from build123d import *

# Parameters (mm, degrees)
F0_R      = 2.7305
F1_DEPTH  = 13.716
F0_W      = 71.12
F0_H      = 39.37
F0_H_2    = 6.35
F2_DEPTH  = 5.08
F3_DEPTH  = 25.4
F4_W      = 43.18
F4_H      = 25.4
F5_DEPTH  = 6.351
F6_R      = 1
F7_DEPTH  = 9
F8_R      = 5.08
F9_W      = 48
F9_H      = 17
F9_W_2    = 11
F9_H_2    = 6.2
F10_DEPTH = 25.4


with BuildPart() as f1:
    # F0 (on Front) → F1 (new body)
    with BuildSketch(Plane.XZ):
        with Locations((6.9215, 40.386)):
            Circle(F0_R)
    extrude(amount=F1_DEPTH)



with BuildPart() as f1b:
    # F0 (on Front) → F1, piece 2 (new body)
    with BuildSketch(Plane.XZ):
        with Locations((6.9215, 10.668)):
            Circle(F0_R)
    extrude(amount=F1_DEPTH)


with BuildPart() as f1c:
    # F0 (on Front) → F1, piece 3 (new body)
    with BuildSketch(Plane.XZ):
        with Locations((64.1985, 10.668)):
            Circle(F0_R)
    extrude(amount=F1_DEPTH)


with BuildPart() as f1d:
    # F0 (on Front) → F1, piece 4 (new body)
    with BuildSketch(Plane.XZ):
        with Locations((64.1985, 40.386)):
            Circle(F0_R)
    extrude(amount=F1_DEPTH)


with BuildPart() as f1_1:
    add(f1.part)

    add(f1b.part)  # F2 merges F1b

    add(f1c.part)  # F2 merges F1c

    add(f1d.part)  # F2 merges F1d
    # F0 (on Front) → F2 (join)
    with BuildSketch(Plane.XZ):
        with Locations((35.56, 26.035)):
            Rectangle(F0_W, F0_H)
        with Locations((6.9215, 10.668)):
            Circle(F0_R, mode=Mode.SUBTRACT)
        with Locations((64.1985, 10.668)):
            Circle(F0_R, mode=Mode.SUBTRACT)
        with Locations((6.9215, 40.386)):
            Circle(F0_R, mode=Mode.SUBTRACT)
        with Locations((64.1985, 40.386)):
            Circle(F0_R, mode=Mode.SUBTRACT)
        with Locations((35.56, 3.175)):
            Rectangle(F0_W, F0_H_2)
        with Locations((64.1985, 40.386)):
            Circle(F0_R)
        with Locations((6.9215, 40.386)):
            Circle(F0_R)
        with Locations((6.9215, 10.668)):
            Circle(F0_R)
        with Locations((64.1985, 10.668)):
            Circle(F0_R)
    extrude(amount=-F2_DEPTH)

    # F0 (on Front) → F3 (join)
    with BuildSketch(Plane.XZ):
        with Locations((35.56, 3.175)):
            Rectangle(F0_W, F0_H_2)
    extrude(amount=F3_DEPTH)

    # F4 (on face) → F5 (cut, through all)
    with BuildSketch(Plane.XY.offset(6.35)):
        with Locations((35.56, -12.7)):
            Rectangle(F4_W, F4_H)
    extrude(amount=-F5_DEPTH, mode=Mode.SUBTRACT)

    # F6 (on face) → F7 (cut)
    with BuildSketch(Plane.XZ.offset(13.716)):
        with Locations((6.9215, 10.668)):
            Circle(F6_R)
        with Locations((6.9215, 40.386)):
            Circle(F6_R)
        with Locations((64.1985, 40.386)):
            Circle(F6_R)
        with Locations((64.1985, 10.668)):
            Circle(F6_R)
    extrude(amount=-F7_DEPTH, mode=Mode.SUBTRACT)

    # F8
    f8_edges = [f1_1.edges().sort_by_distance(p)[0] for p in [
        (0, 2.54, 45.72),
        (71.12, 2.54, 45.72),
    ]]
    fillet(f8_edges, radius=F8_R)

    # F9 (on face) → F10 (cut)
    with BuildSketch(Plane(origin=(0, 5.08, 0), x_dir=(-1, 0, 0), z_dir=(0, 1, 0))):
        with Locations((-35.56, 37.22)):
            Rectangle(F9_W, F9_H)
        with Locations((-35.56, 10.32)):
            Rectangle(F9_W_2, F9_H_2)
    extrude(amount=-F10_DEPTH, mode=Mode.SUBTRACT)


solid = f1_1.part
Source: CAD feature listing. Evaluate the final solid. Frame: model axes, mm. A direction names the side the tool comes from. Give positions to 0.01 mm unless a question says otherwise; leave off trailing zeros. Order: outer loops, then holes, each group sorted by start corner. A loop starts at its lowest first (then second) coordinate and runs counter-clockwise, first axis right, second up. Notation, with made-up numbers: (77.5, 31.5) -> (127.5, 31.5) arc R10 ccw to (127.5, 35.5) -> close; hole circle Ø2 at (-18, 49.25). An arc over 180 degrees is marked (long way). Use a Markdown table: item, result.
1) Ray query, line 1 along X through (y, z) = (-8.5, 4); line 2 along Z through (x, y) = (6.5, -12.5); line 3 along Y through (x, z) = (44.5, 13). Return the intervals inside material, ascending. Write a range as [from, to].
Answer list:
| item | result |
|---|---|
| line 1 | [0, 13.97], [57.15, 71.12] |
| line 2 | [0, 6.35], [7.97, 9.76], [11.57, 13.37], [37.69, 39.48], [41.29, 43.08] |
| line 3 | [0, 5.08] |
2) Contact query for flat-ended pins moving along their axis: P1, Ø4.5, axis at x = 7, z = 9.5, coming from the -Y side; P2, Ø12, axis at x = 33.5, y = 0, coming from the +Z side; P3, Ø8, axis at x = 44, z = 6.5, coming from the -Y side; P4, Ø12, axis at y = -17, z = 20, coming from the -X side. Output: stop coordinate, or through.
Answer list:
| item | result |
|---|---|
| P1 | y = -13.72 |
| P2 | z = 28.72 |
| P3 | y = 0 |
| P4 | through |
3) Section query C-C, the plane z = 5. Return the cut outline in (x, y), then the cut area to 3 significant figures.
Answer list:
| item | result |
|---|---|
| outline | (0, -25.4) -> (13.97, -25.4) -> (13.97, 0) -> (57.15, 0) -> (57.15, -25.4) -> (71.12, -25.4) -> (71.12, 5.08) -> (0, 5.08) -> close |
| area | 1,070 mm² |
4) Section query A-A, the plane y = -23. Return the cut outline in (x, z), then the cut area to 3 significant figures.
Answer list:
| item | result |
|---|---|
| outline | (0, 0) -> (13.97, 0) -> (13.97, 6.35) -> (0, 6.35) -> close; (57.15, 0) -> (71.12, 0) -> (71.12, 6.35) -> (57.15, 6.35) -> close |
| area | 177 mm² |
5) Mould query, pull axis X, two halves, no side actions, for faces 1 (the cylindrical face through (1.449, 2.576, 44.192)), 2 (the flat face through (63, 3, 45.72)), 3 (the flat face through (64, -4.716, 11)). Classes: +X half, -X half, draft (parallel to the pull), parting line (faces both ways), or undercut.
Answer list:
| item | result |
|---|---|
| face 1 | -X half |
| face 2 | draft |
| face 3 | undercut |
6) Section query D-D, the plane y = -1. Return the cut outline in (x, z), then the cut area to 3 significant figures.
Answer list:
| item | result |
|---|---|
| outline | (0, 0) -> (13.97, 0) -> (13.97, 6.35) -> (0, 6.35) -> close; circle Ø5.46 at (6.92, 10.67); circle Ø5.46 at (6.92, 40.39); (57.15, 0) -> (71.12, 0) -> (71.12, 6.35) -> (57.15, 6.35) -> close; circle Ø5.46 at (64.2, 10.67); circle Ø5.46 at (64.2, 40.39) |
| area | 271 mm² |
7) Section query B-B, the plane x = 33. Return the cut outline in (y, z).
Answer list:
| item | result |
|---|---|
| outline | (0, 0) -> (5.08, 0) -> (5.08, 7.22) -> (0, 7.22) -> close; (0, 13.42) -> (5.08, 13.42) -> (5.08, 28.72) -> (0, 28.72) -> close |
8) Reachability of faces 4 (the flat face through (65.4, -13.716, 10.7)), 5 (the flat face through (36, 3, 13.42)), 6 (the cylindrical face through (65.458, -6.762, 8.246)) from +Z, -Z, +X, -X, +Y, -Y: full face, straight path, thin tool, end or side. Return the list, or none.
Answer list:
| item | result |
|---|---|
| face 4 | +Z, +X, -X, -Y |
| face 5 | +Y, -Y |
| face 6 | -Y |
